For this review, take the finished solid that the model builds, in its own axes (mm). Face numbers are marked on the shaded views. A direction names the side the tool comes from. Coordinates: 2 decimals unless noted, no trailing zeros. Write each loop counter-clockwise with the first axis right and the second up, starting at its lowest first coordinate (ties: lowest second). Pieces come first, ordered by that corner, then holes.
1) To check wall thickness, follow line 1 along X through (y, z) = (-6, 4); line 2 along X through (y, z) = (33, 1.75); line 3 along Y through (x, z) = (2.5, 8.5). State the ranges of each line that lie inside material, in increasing order.
2) We need section A-A on y = -42. Write out the cut boundary in (x, z).
3) We need section B-B on x = 27. Write out the cut boundary in (y, z), then the cut area to 3 significant figures.
4) For the marked faces 1 and 2, list the 3-axis set-ups (+Z, -Z, +X, -X, +Y, -Y) from which the entire face can be reached by the end or side of a thin tool; tool diameter is ignored.
5) Mouldability with a two-part tool opening along Y and no side actions: class the marked faces 3, 4 and 5 as pulls with the +Y half, pulls with the -Y half, needs draft (parallel to the pull), parting line crosses it, or undercut.
6) We need section C-C on z = 3. Write out the cut boundary in (x, y).
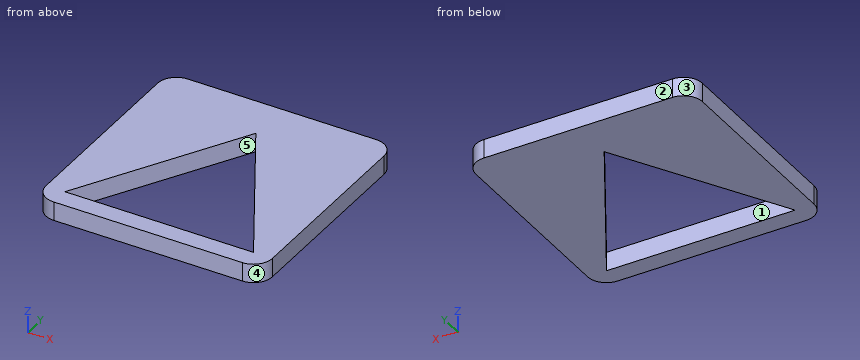
from build123d import *

# Parameters (mm, degrees)
BOSS_EXTRUDE1_DEPTH = 10
CUT_EXTRUDE1_DEPTH  = 10


with BuildPart() as part:
    # Sketch1 → Boss-Extrude1 (new body)
    with BuildSketch(Plane.XY):
        with BuildLine():
            Line((-50, 60), (50, 60))
            ThreePointArc((50, 60), (57.071067812, 57.071067812), (60, 50))
            Line((60, 50), (60, -50))
            ThreePointArc((60, -50), (57.071067812, -57.071067812), (50, -60))
            Line((50, -60), (-50, -60))
            ThreePointArc((-50, -60), (-57.071067812, -57.071067812), (-60, -50))
            Line((-60, -50), (-60, 50))
            ThreePointArc((-60, 50), (-57.071067812, 57.071067812), (-50, 60))
        make_face()
    extrude(amount=BOSS_EXTRUDE1_DEPTH)

    # Sketch3 → Cut-Extrude1 (cut)
    with BuildSketch(Plane.XY.offset(10)):
        Polygon((-50, -50), (50, -50), (0, 36.602540378), align=None)
    extrude(amount=-CUT_EXTRUDE1_DEPTH, mode=Mode.SUBTRACT)


solid = part.part
Result:
1. line 1: x = -60 to -24.6, 24.6 to 60
1. line 2: x = -60 to -2.08, 2.08 to 60
1. line 3: y = -60 to -50, 32.27 to 60
2. outline: (-60, 0) - (-45.38, 0) - (-45.38, 10) - (-60, 10) - close; (45.38, 0) - (60, 0) - (60, 10) - (45.38, 10) - close
3. outline: (-60, 0) - (-50, 0) - (-50, 10) - (-60, 10) - close; (-10.16, 0) - (60, 0) - (60, 10) - (-10.16, 10) - close
3. area: 802 mm2
4. face 1: +Z, -Z
4. face 2: +Z, -Z, +X, -X, +Y
5. face 3: pulls with the +Y half
5. face 4: pulls with the -Y half
5. face 5: undercut
6. outline: (-60, -50) arc R10 ccw to (-50, -60) - (50, -60) arc R10 ccw to (60, -50) - (60, 50) arc R10 ccw to (50, 60) - (-50, 60) arc R10 ccw to (-60, 50) - close; hole (-50, -50) - (50, -50) - (0, 36.6) - close
